Source: CAD feature listing. Evaluate the final solid. Frame: model axes, mm. Give positions to 0.01 mm unless a question says otherwise; leave off trailing zeros. Order: outer loops, then holes, each group sorted by start corner. A loop starts at its lowest first (then second) coordinate and runs counter-clockwise, first axis right, second up. Notation, with made-up numbers: (79.25, 74) - (137.25, 74) arc R21 cw to (137.25, 106) - close; hole circle Ø6 at (-11.75, 80). An arc over 180 degrees is marked (long way). Write each question's results on one line, items separated by ' | '. Start each with the question number.
Item 1: Section B-B on x = -1.75. Output: boundary loops of the cut face in (y, z) (1 decimal), and give its area (3 significant figures).
Item 2: Line query: line 1 along Z through (x, y) = (-3, -4) (1 decimal); line 2 along Y through (x, z) = (1.5, 286); line 3 along Y through (x, z) = (1, 818). Output: solid intervals per line, ascending.
Item 3: Section A-A on z = 210. Output: boundary loops of the cut face in (x, y).
Item 4: Contact query for flat-ended pins moving along their axis: pin 1 Ø4 at (x, y) = (2, 2.5) entering from -Z; pin 2 Ø1 at (y, z) = (1.5, 599.5) entering from +X; pin 3 Ø3 at (x, z) = (3, 596.5) entering from -Y; pin 4 Ø5 at (y, z) = (-4, 380) entering from -X. Output: stop coordinate, or through.
```python
from build123d import *

# Parameters (mm, degrees)
SKETCH1_R           = 6.35
BOSS_EXTRUDE1_DEPTH = 914.4
SKETCH3_R           = 6.35
SKETCH3_R_2         = 3.96875
CUT_EXTRUDE1_DEPTH  = 7.9375
SKETCH4_R           = 6.35
SKETCH4_R_2         = 3.96875
CUT_EXTRUDE2_DEPTH  = 7.9375


with BuildPart() as part:
    # Sketch1 → Boss-Extrude1 (new body)
    with BuildSketch(Plane.XY):
        Circle(SKETCH1_R)
    extrude(amount=BOSS_EXTRUDE1_DEPTH)

    # Sketch3 → Cut-Extrude1 (cut)
    with BuildSketch(Plane(origin=(0, 0, 50.8), x_dir=(-1, 0, 0), z_dir=(0, 0, -1))):
        Circle(SKETCH3_R)
        Circle(SKETCH3_R_2, mode=Mode.SUBTRACT)
    extrude(amount=-CUT_EXTRUDE1_DEPTH, mode=Mode.SUBTRACT)

    # Sketch4 → Cut-Extrude2 (cut)
    with BuildSketch(Plane(origin=(0, 0, 344.4875), x_dir=(-1, 0, 0), z_dir=(0, 0, -1))):
        Circle(SKETCH4_R)
        Circle(SKETCH4_R_2, mode=Mode.SUBTRACT)
    extrude(amount=-CUT_EXTRUDE2_DEPTH, mode=Mode.SUBTRACT)


solid = part.part
```
Evaluation:
1) outline: (-6.1, 0) - (6.1, 0) - (6.1, 50.8) - (3.6, 50.8) - (3.6, 58.7) - (6.1, 58.7) - (6.1, 344.5) - (3.6, 344.5) - (3.6, 352.4) - (6.1, 352.4) - (6.1, 914.4) - (-6.1, 914.4) - (-6.1, 352.4) - (-3.6, 352.4) - (-3.6, 344.5) - (-6.1, 344.5) - (-6.1, 58.7) - (-3.6, 58.7) - (-3.6, 50.8) - (-6.1, 50.8) - close | area: 11,100 mm^2
2) line 1: z = 0 to 50.8, 58.7 to 344.5, 352.4 to 914.4 | line 2: y = -6.17 to 6.17 | line 3: y = -6.27 to 6.27
3) outline: circle Ø12.7 at (0, 0)
4) pin 1: stops at z = 0 | pin 2: stops at x = 6.27 | pin 3: stops at y = -6.17 | pin 4: stops at x = -6.17
